Geometry check sheet. Reference: the model listing, model coordinates, mm. Coordinates: 2 decimals unless noted, no trailing zeros.
```python
from build123d import *

# Parameters (mm, degrees)
SKETCH_9_R          = 4
CUT_EXTRUDE_3_DEPTH = 0.5


with BuildPart() as part:
    # 草图2 → 旋转1 (revolve)
    with BuildSketch(Plane.XY):
        with BuildLine():
            Line((0, 28), (0, -28))
            add(Edge.make_bspline(
                [(0, -28), (30, -28), (30, 0), (30, 28), (0, 28)],
                knots=[4.71238898, 4.71238898, 4.71238898, 6.283185307, 6.283185307, 7.853981634, 7.853981634, 7.853981634], degree=2, weights=[1, 0.707106781, 1, 0.707106781, 1]))
        make_face()
    revolve(axis=Axis((0, 28, 0), (0, -1, 0)))

    # 草图9 → 切除-拉伸3 (cut)
    with BuildSketch(Plane(origin=(0, 28, 0), x_dir=(1, 0, 0), z_dir=(0, 1, 0))):
        with Locations(Location((0, 0, 0), (0, 0, 270))):
            Circle(SKETCH_9_R)
    extrude(amount=-CUT_EXTRUDE_3_DEPTH, mode=Mode.SUBTRACT)

    # 草图10 → 旋转2 (revolve)
    with BuildSketch(Plane.XY, mode=Mode.PRIVATE) as revolve_2_sk:
        with BuildLine():
            Line((0, 27.5), (3, 27.5))
            add(Edge.make_bspline(
                [(2, 31), (1.428667746, 28.919998941), (3, 27.5)],
                knots=[0, 0, 0, 1, 1, 1], degree=2))
            Line((2, 31), (2.5, 31))
            Line((2.5, 31), (2.5, 32.5))
            Line((2.5, 32.5), (0, 32.5))
            Line((0, 32.5), (0, 27.5))
        make_face()
    revolve(revolve_2_sk.sketch.rotate(Axis((0, 27.5, 0), (0, 1, 0)), 90), axis=Axis((0, 27.5, 0), (0, 1, 0)))

    # 草图11 → 切除-旋转1 (revolve, cut)
    with BuildSketch(Plane.XY):
        with BuildLine():
            Line((0, 20), (0, -20))
            ThreePointArc((0, -20), (20, 0), (0, 20))
        make_face()
    revolve(axis=Axis((0, 20, 0), (0, -1, 0)), mode=Mode.SUBTRACT)


solid = part.part
```
Item 1: Depth check by flat-ended pin: P1, Ø1, axis at x = 11.5, z = -18.5, coming from the -Y side; P2, Ø6, axis at x = 17, y = -15, coming from the -Z side; P3, Ø2, axis at x = -11, y = 18, coming from the -Z side; P4, Ø2.5, axis at x = 0, z = -0.5, coming from the -Y side. Enter the tip coordinate at first touch or a pass-through.
Item 2: Release check for a two-part mould opening along Z. For faces 1 (the face through (-2, 31, -1)), 2 (the face through (-0.1, 31.8, 2.5)), 3 (the face through (3, 27.5, 1)) record: pulls with the +Z half, pulls with the -Z half, needs draft (parallel to the pull), parting line crosses it, or undercut.
Item 3: Thickness scan on line 1 along Z through (x, y) = (-5.5, -12); line 2 along X through (y, z) = (-13, 8); line 3 along Z through (x, y) = (7, -7). Record the ranges inside material, lowest first.
Geometry check:
1. P1: stops at y = -19.73
1. P2: stops at z = -22.1
1. P3: stops at z = -21.28
1. P4: stops at y = -28
2. face 1: needs draft
2. face 2: parting line crosses it
2. face 3: undercut
3. line 1: z = -26.54 to -15.02, 15.02 to 26.54
3. line 2: x = -25.34 to -12.92, 12.92 to 25.34
3. line 3: z = -28.19 to -17.38, 17.38 to 28.19
